```python
from build123d import *

# Parameters (mm, degrees)
SKETCH2_W           = 20
SKETCH2_H           = 70
BOSS_EXTRUDE1_DEPTH = 20
SKETCH3_W           = 9.5
SKETCH3_H           = 70
CUT_EXTRUDE1_DEPTH  = 0.5
SKETCH4_R           = 2.35
CUT_EXTRUDE2_DEPTH  = 5.5
SKETCH5_W           = 20
SKETCH5_H           = 20
BOSS_EXTRUDE2_DEPTH = 5
FILLET1_R           = 6
FILLET2_R           = 6
SKETCH6_W           = 60
SKETCH6_H           = 5.5
BOSS_EXTRUDE3_DEPTH = 1
CHAMFER1_SIZE       = 1
SKETCH7_R           = 2.625
CUT_EXTRUDE3_DEPTH  = 75.520767082
FILLET3_R           = 5
FILLET4_R           = 5


with BuildPart() as part:
    # Sketch2 → Boss-Extrude1 (new body)
    with BuildSketch(Plane.XY):
        with Locations((-0.46875, 8.59375)):
            Rectangle(SKETCH2_W, SKETCH2_H)
    extrude(amount=BOSS_EXTRUDE1_DEPTH)

    # Sketch3 → Cut-Extrude1 (cut)
    with BuildSketch(Plane.XY.offset(20)):
        with Locations((-0.46875, 8.59375)):
            Rectangle(SKETCH3_W, SKETCH3_H)
    extrude(amount=-CUT_EXTRUDE1_DEPTH, mode=Mode.SUBTRACT)

    # Sketch4 → Cut-Extrude2 (cut)
    with BuildSketch(Plane.XY.offset(19.5)):
        with Locations((-0.46875, 38.59375)):
            Circle(SKETCH4_R)
        with Locations((-0.46875, 18.59375)):
            Circle(SKETCH4_R)
        with Locations((-0.46875, -1.40625)):
            Circle(SKETCH4_R)
        with Locations((-0.46875, 78.59375)):
            Circle(SKETCH4_R)
        with Locations((-0.46875, -21.40625)):
            Circle(SKETCH4_R)
        with Locations((-0.46875, 58.59375)):
            Circle(SKETCH4_R)
    extrude(amount=-CUT_EXTRUDE2_DEPTH, mode=Mode.SUBTRACT)

    # Sketch5 → Boss-Extrude2 (add)
    with BuildSketch(Plane(origin=(0, 43.59375, 0), x_dir=(1, 0, 0), z_dir=(0, 1, 0))):
        with Locations((19.53125, -10)):
            Rectangle(SKETCH5_W, SKETCH5_H)
        with Locations((-20.46875, -10)):
            Rectangle(SKETCH5_W, SKETCH5_H)
    extrude(amount=-BOSS_EXTRUDE2_DEPTH)

    # Fillet1
    fillet1_edges = [part.edges().sort_by_distance(p)[0] for p in [
        (9.53125, 38.59375, 10),
    ]]
    fillet(fillet1_edges, radius=FILLET1_R)

    # Fillet2
    fillet2_edges = [part.edges().sort_by_distance(p)[0] for p in [
        (-10.46875, 38.59375, 10),
    ]]
    fillet(fillet2_edges, radius=FILLET2_R)

    # Sketch6 → Boss-Extrude3 (add)
    with BuildSketch(Plane(origin=(0, 43.59375, 0), x_dir=(1, 0, 0), z_dir=(0, 1, 0))):
        with Locations((-0.46875, -10)):
            Rectangle(SKETCH6_W, SKETCH6_H)
    extrude(amount=BOSS_EXTRUDE3_DEPTH)

    # Chamfer1
    chamfer1_edges = [part.edges().sort_by_distance(p)[0] for p in [
        (-0.46875, 44.59375, 7.25),
        (-0.46875, 44.59375, 12.75),
    ]]
    chamfer(chamfer1_edges, length=CHAMFER1_SIZE - 0.0001)  # a hair under: the kernel refuses the full size

    # Sketch7 → Cut-Extrude3 (cut, through all)
    with BuildSketch(Plane.XZ.offset(-38.59375)):
        with Locations(Location((19.53125, 10, 0), (0, 0, 270))):
            Circle(SKETCH7_R)
        with Locations(Location((-20.46875, 10, 0), (0, 0, 270))):
            Circle(SKETCH7_R)
    extrude(amount=-CUT_EXTRUDE3_DEPTH, mode=Mode.SUBTRACT)

    # Fillet3
    fillet3_edges = [part.edges().sort_by_distance(p)[0] for p in [
        (-10.46875, -26.40625, 10),
    ]]
    fillet(fillet3_edges, radius=FILLET3_R)

    # Fillet4
    fillet4_edges = [part.edges().sort_by_distance(p)[0] for p in [
        (9.53125, -26.40625, 10),
    ]]
    fillet(fillet4_edges, radius=FILLET4_R)


solid = part.part
```
Work out the finished part from the listing and answer in its coordinate system (mm). A direction names the side the tool comes from. Give positions to 0.01 mm unless a question says otherwise; leave off trailing zeros. Order: outer loops, then holes, each group sorted by start corner. A loop starts at its lowest first (then second) coordinate and runs counter-clockwise, first axis right, second up. Notation, with made-up numbers: (70, 36.25) - (129, 36.25) arc R28 cw to (129, 65.25) - close; hole circle Ø5 at (44, 20). An arc over 180 degrees is marked (long way). One line per item, written item: value. Start each with the question number.
1. Section A-A, the plane z = 10 is taken. Write down the section's boundary in (x, y).
2. Each of these flat-tipped pins is pushed along its axis until it touches: pin 1 Ø1.4 at (x, y) = (-0.5, 17.5) entering from +Z; pin 2 Ø8 at (y, z) = (23, 11) entering from -X; pin 3 Ø8 at (x, z) = (-3.5, 2.5) entering from +Y. Where does it stop, or does it pass through?
3. Section C-C, the plane z = 4 is taken. Write down the section's boundary in (x, y).
4. Consider line 1 (X direction, y = 41.3, z = 10); line 2 (Y direction, x = 17.5, z = 1.75); line 3 (Y direction, x = 23, z = 11.5). Determine where each line is inside the solid, lowest interval first.
5. Which of the six approach directions +Z, -Z, +X, -X, +Y, -Y give full straight-line access (tool end or side, diameter ignored) to faces 1 (the face through (-10.469, 5, 10)), 2 (the face through (-2.33, -2.84, 16.79)), 3 (the face through (9.531, 5, 10)), 4 (the face through (-1, 43.594, 16))?
6. For a pull along X with two mould halves and no side action, classify faces 5 (the face through (-9.043, -24.903, 10.14)), 6 (the face through (-1, 9, 19.5)), 7 (the face through (-24, 38.594, 10)), 8 (the face through (-1, 39, 14)) as released by +X, released by -X, zero draft, split by the parting line, or undercut.
7. Section B-B, the plane y = 22 is taken. Write down the section's boundary in (x, z), then the cut area to 3 significant figures.
Filled sheet:
1. outline: (-30.47, 38.59) - (-23.09, 38.59) - (-23.09, 44.59) - (-30.47, 44.59) - close; (-17.84, 38.59) - (-16.47, 38.59) arc R6 cw to (-10.47, 32.59) - (-10.47, -21.41) arc R5 ccw to (-5.47, -26.41) - (4.53, -26.41) arc R5 ccw to (9.53, -21.41) - (9.53, 32.59) arc R6 cw to (15.53, 38.59) - (16.91, 38.59) - (16.91, 44.59) - (-17.84, 44.59) - close; (22.16, 38.59) - (29.53, 38.59) - (29.53, 44.59) - (22.16, 44.59) - close
2. pin 1: z = 14
2. pin 2: x = -10.47
2. pin 3: y = 43.59
3. outline: (-30.47, 38.59) - (-16.47, 38.59) arc R6 cw to (-10.47, 32.59) - (-10.47, -21.41) arc R5 ccw to (-5.47, -26.41) - (4.53, -26.41) arc R5 ccw to (9.53, -21.41) - (9.53, 32.59) arc R6 cw to (15.53, 38.59) - (29.53, 38.59) - (29.53, 43.59) - (-30.47, 43.59) - close
4. line 1: -30.47 to -23.09, -17.84 to 16.91, 22.16 to 29.53
4. line 2: 38.59 to 43.59
4. line 3: 38.59 to 44.59
5. face 1: +Z, -Z, -X, -Y
5. face 2: +Z
5. face 3: +Z, -Z, +X, -Y
5. face 4: +Z, +X, -X, +Y
6. face 5: released by -X
6. face 6: undercut
6. face 7: zero draft
6. face 8: undercut
7. outline: (-10.47, 0) - (9.53, 0) - (9.53, 20) - (4.28, 20) - (4.28, 19.5) - (-5.22, 19.5) - (-5.22, 20) - (-10.47, 20) - close
7. area: 395 mm²
